```python
from build123d import *

# Parameters (mm, degrees)
SKETCH_1_R      = 2
EXTRUDE_2_DEPTH = 2


with BuildPart() as part:
    # 草图1 → 凸台-拉伸2 (new body)
    with BuildSketch(Plane.XY):
        with BuildLine():
            Line((-29.994433528, 12.494433528), (-25.48340173, 12.494433528))
            ThreePointArc((-25.48340173, 12.494433528), (-13.947547573, 15.894235428), (-2, 17.269259451))
            Line((-2, 17.269259451), (-2, 13.53))
            ThreePointArc((-2, 13.53), (0, 11.53), (2, 13.53))
            Line((2, 13.53), (2, 17.269259451))
            ThreePointArc((2, 17.269259451), (13.947547573, 15.894235428), (25.48340173, 12.494433528))
            Line((25.48340173, 12.494433528), (29.994433528, 12.494433528))
            Line((29.994433528, 12.494433528), (29.994433528, 14.494433528))
            Line((29.994433528, 14.494433528), (37, 14.494433528))
            Line((37, 14.494433528), (37, 12.5))
            Line((37, 12.5), (41, 12.5))
            Line((41, 12.5), (41, 9.3))
            Line((41, 9.3), (43, 9.3))
            Line((43, 9.3), (43, 4.3))
            Line((43, 4.3), (41, 4.3))
            Line((41, 4.3), (41, 1.5))
            Line((41, 1.5), (38.5, 1.5))
            Line((38.5, 1.5), (38.5, 3))
            Line((38.5, 3), (35.9, 3))
            Line((35.9, 3), (35.9, 1.5))
            Line((35.9, 1.5), (32.9, 1.5))
            Line((32.9, 1.5), (32.9, -1.5))
            Line((32.9, -1.5), (35.9, -1.5))
            Line((35.9, -1.5), (35.9, -3))
            Line((35.9, -3), (38.5, -3))
            Line((38.5, -3), (38.5, -1.5))
            Line((38.5, -1.5), (41, -1.5))
            Line((41, -1.5), (41, -4.3))
            Line((41, -4.3), (43, -4.3))
            Line((43, -4.3), (43, -9.3))
            Line((43, -9.3), (41, -9.3))
            Line((41, -9.3), (41, -12.5))
            Line((41, -12.5), (37, -12.5))
            Line((37, -12.5), (37, -14.5))
            Line((37, -14.5), (30, -14.5))
            Line((30, -14.5), (30, -12.485627756))
            Line((30, -12.485627756), (25.50333236, -12.485627756))
            ThreePointArc((25.50333236, -12.485627756), (22.164855453, -13.695011333), (18.769346851, -14.733547814))
            Line((18.769346851, -14.733547814), (13.437476273, -5.744669088))
            ThreePointArc((13.437476273, -5.744669088), (10.696992802, -5.04484744), (9.997171153, -7.785330912))
            Line((9.997171153, -7.785330912), (14.711679138, -15.733412155))
            ThreePointArc((14.711679138, -15.733412155), (0.337099689, -17.296013049), (-14.051862928, -15.871930634))
            Line((-14.051862928, -15.871930634), (-9.997171153, -7.785330912))
            ThreePointArc((-9.997171153, -7.785330912), (-10.696992802, -5.04484744), (-13.437476273, -5.744669088))
            Line((-13.437476273, -5.744669088), (-18.769346851, -14.733547814))
            ThreePointArc((-18.769346851, -14.733547814), (-22.164855453, -13.695011333), (-25.50333236, -12.485627756))
            Line((-25.50333236, -12.485627756), (-30, -12.485627756))
            Line((-30, -12.485627756), (-30, -14.5))
            Line((-30, -14.5), (-37, -14.5))
            Line((-37, -14.5), (-37, -12.5))
            Line((-37, -12.5), (-41, -12.5))
            Line((-41, -12.5), (-41, -9.3))
            Line((-41, -9.3), (-43, -9.3))
            Line((-43, -9.3), (-43, -4.3))
            Line((-43, -4.3), (-41, -4.3))
            Line((-41, -4.3), (-41, -1.5))
            Line((-41, -1.5), (-38.5, -1.5))
            Line((-38.5, -1.5), (-38.5, -3))
            Line((-38.5, -3), (-35.9, -3))
            Line((-35.9, -3), (-35.9, -1.5))
            Line((-35.9, -1.5), (-32.9, -1.5))
            Line((-32.9, -1.5), (-32.9, 1.5))
            Line((-32.9, 1.5), (-35.9, 1.5))
            Line((-35.9, 1.5), (-35.9, 3))
            Line((-35.9, 3), (-38.5, 3))
            Line((-38.5, 3), (-38.5, 1.5))
            Line((-38.5, 1.5), (-41, 1.5))
            Line((-41, 1.5), (-41, 4.3))
            Line((-41, 4.3), (-43, 4.3))
            Line((-43, 4.3), (-43, 9.3))
            Line((-43, 9.3), (-41, 9.3))
            Line((-41, 9.3), (-41, 12.5))
            Line((-41, 12.5), (-37, 12.5))
            Line((-37, 12.5), (-37, 14.494433528))
            Line((-37, 14.494433528), (-29.994433528, 14.494433528))
            Line((-29.994433528, 14.494433528), (-29.994433528, 12.494433528))
        make_face()
        Circle(SKETCH_1_R, mode=Mode.SUBTRACT)
    extrude(amount=EXTRUDE_2_DEPTH)


solid = part.part
```
The model under review builds one solid part; all positions refer to its coordinate system, in mm. A direction names the side the tool comes from. Round coordinates to 2 decimals unless told otherwise and drop trailing zeros. Write each loop counter-clockwise with the first axis right and the second up, starting at its lowest first coordinate (ties: lowest second). Pieces come first, ordered by that corner, then holes. Notation, with made-up numbers: M 28.25,71.25 L 57.25,71.25 A24 cw 57.25,92.25 Z; hole C 7,-16 d10. An arc over 180 degrees is marked long. Use CSV: the item, a comma, the result in double quotes. Start each with the question number.
(1) For line 1 along Y through (x, z) = (-35, 0.7); line 2 along Y through (x, z) = (0, 0.7); line 3 along Y through (x, z) = (26.5, 0.75), list the stretches that pass through material, from the lowest coordinate up.
(2) We need section B-B, the plane x = 0. State the section outline as (y, z) points.
(3) Tool access review of faces 1 (the face through (16.14, -10.3, 0.99)), 2 (the face through (-33, -14.5, 1)), 3 (the face through (-28, -12.486, 1)), 4 (the face through (34, -1.5, 1)), 5 (the face through (13.78, 15.93, 0.99)): name each direction out of +Z, -Z, +X, -X, +Y, -Y from which nothing blocks a thin tool from reaching the whole face with its end or side.
(4) We need section A-A, the plane y = 0. State the section outline as (x, z) points.
(5) Clearance check with flat-ended pins moving along their axes: P1, Ø1, axis at x = 35, z = 1.5, coming from the +Y side; P2, Ø1, axis at x = -19, z = 1, coming from the -Y side. State where each tip first meets the part, or that it passes through.
(6) The part is to be moulded in two halves that separate along X. For faces 6 (the face through (-43, -7, 1)), 7 (the face through (1, -4, 2)), 8 (the face through (-38.5, -2, 1)), 9 (the face through (41, -3, 1)), say which applies: +X half, -X half, draft (parallel to the pull), parting line (faces both ways), or undercut.
Findings:
1,line 1,"-14.5 to -1.5, 1.5 to 14.49"
1,line 2,"-17.3 to -2, 2 to 11.53"
1,line 3,"-12.49 to 12.49"
2,outline,"M -17.3,0 L -2,0 L -2,2 L -17.3,2 Z; M 2,0 L 11.53,0 L 11.53,2 L 2,2 Z"
3,face 1,"+Z, -Z"
3,face 2,"+Z, -Z, -X, -Y"
3,face 3,"+Z, -Z, -Y"
3,face 4,"+Z, -Z, +X"
3,face 5,"+Z, -Z, +Y"
4,outline,"M -32.9,0 L -2,0 L -2,2 L -32.9,2 Z; M 2,0 L 32.9,0 L 32.9,2 L 2,2 Z"
5,P1,"y = 14.49"
5,P2,"y = -14.73"
6,face 6,"-X half"
6,face 7,"draft"
6,face 8,"undercut"
6,face 9,"+X half"
